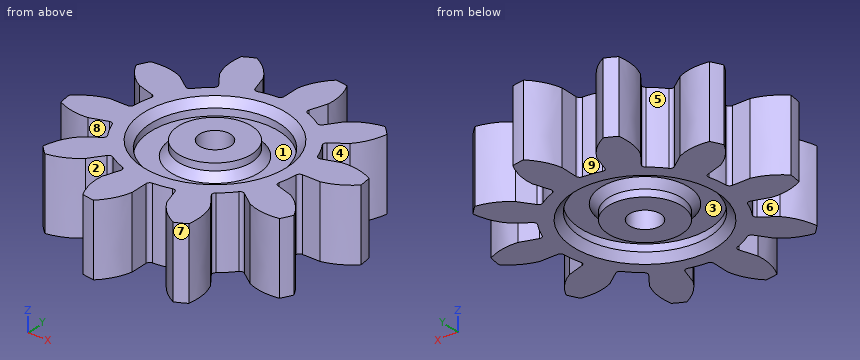
```python
from build123d import *

# Parameters (mm, degrees)
BOSS_EXTRUDE1_DEPTH = 10
CIRPATTERN1_COUNT   = 10
SKETCH1_R           = 11.7825
BOSS_EXTRUDE2_DEPTH = 10
SKETCH4_R           = 8.946052481
SKETCH4_R_2         = 5.101265003
CUT_EXTRUDE1_DEPTH  = 2
SKETCH4_3_R         = 2.163600103
CUT_EXTRUDE2_DEPTH  = 11.0000001
SKETCH5_R           = 8.946052481
SKETCH5_R_2         = 5.101265003
CUT_EXTRUDE3_DEPTH  = 2
FILLET1_R           = 0.5
CHAMFER1_SIZE       = 1
CHAMFER2_SIZE       = 1


with BuildPart() as part:
    # Sketch3 → Boss-Extrude1 (new body)
    with BuildSketch(Plane.XY):
        with BuildLine():
            Line((4.803075617, 13.959368513), (3.833494733, 11.141437267))
            ThreePointArc((3.833494733, 11.141437267), (1.943363276, 11.621129266), (0, 11.7825))
            Line((0, 11.7825), (0, 14.762571073))
            add(Edge.make_bspline(
                [(0, 14.762571073), (0.333518774, 16.315241106), (1.140884964, 17.626707575), (2.241097954, 18.718316804)],
                knots=[0, 0, 0, 0, 0.256830749, 0.256830749, 0.256830749, 0.256830749], degree=3))
            ThreePointArc((2.241097954, 18.718316804), (3.109381242, 18.593806826), (3.970932877, 18.429042191))
            add(Edge.make_bspline(
                [(4.803075617, 13.959368513), (4.992871831, 15.536072798), (4.656124965, 17.038865536), (3.970932877, 18.429042191)],
                knots=[0, 0, 0, 0, 0.256830749, 0.256830749, 0.256830749, 0.256830749], degree=3))
        make_face()
    extrude(amount=BOSS_EXTRUDE1_DEPTH)


with BuildPart() as cirpattern1_1:
    # CirPattern1: pattern copy
    add(part.part.rotate(Axis((0, 0, 0), (0, 0, 1)), 1 * 360 / CIRPATTERN1_COUNT))


with BuildPart() as cirpattern1_2:
    # CirPattern1: pattern copy
    add(part.part.rotate(Axis((0, 0, 0), (0, 0, 1)), 2 * 360 / CIRPATTERN1_COUNT))


with BuildPart() as cirpattern1_3:
    # CirPattern1: pattern copy
    add(part.part.rotate(Axis((0, 0, 0), (0, 0, 1)), 3 * 360 / CIRPATTERN1_COUNT))


with BuildPart() as cirpattern1_4:
    # CirPattern1: pattern copy
    add(part.part.rotate(Axis((0, 0, 0), (0, 0, 1)), 4 * 360 / CIRPATTERN1_COUNT))


with BuildPart() as cirpattern1_5:
    # CirPattern1: pattern copy
    add(part.part.rotate(Axis((0, 0, 0), (0, 0, 1)), 5 * 360 / CIRPATTERN1_COUNT))


with BuildPart() as cirpattern1_6:
    # CirPattern1: pattern copy
    add(part.part.rotate(Axis((0, 0, 0), (0, 0, 1)), 6 * 360 / CIRPATTERN1_COUNT))


with BuildPart() as cirpattern1_7:
    # CirPattern1: pattern copy
    add(part.part.rotate(Axis((0, 0, 0), (0, 0, 1)), 7 * 360 / CIRPATTERN1_COUNT))


with BuildPart() as cirpattern1_8:
    # CirPattern1: pattern copy
    add(part.part.rotate(Axis((0, 0, 0), (0, 0, 1)), 8 * 360 / CIRPATTERN1_COUNT))


with BuildPart() as cirpattern1_9:
    # CirPattern1: pattern copy
    add(part.part.rotate(Axis((0, 0, 0), (0, 0, 1)), 9 * 360 / CIRPATTERN1_COUNT))


with BuildPart() as part_1:
    add(part.part)

    add(cirpattern1_1.part)  # Boss-Extrude2 merges CirPattern1_1

    add(cirpattern1_2.part)  # Boss-Extrude2 merges CirPattern1_2

    add(cirpattern1_3.part)  # Boss-Extrude2 merges CirPattern1_3

    add(cirpattern1_4.part)  # Boss-Extrude2 merges CirPattern1_4

    add(cirpattern1_5.part)  # Boss-Extrude2 merges CirPattern1_5

    add(cirpattern1_6.part)  # Boss-Extrude2 merges CirPattern1_6

    add(cirpattern1_7.part)  # Boss-Extrude2 merges CirPattern1_7

    add(cirpattern1_8.part)  # Boss-Extrude2 merges CirPattern1_8

    add(cirpattern1_9.part)  # Boss-Extrude2 merges CirPattern1_9
    # Sketch1 → Boss-Extrude2 (add)
    with BuildSketch(Plane.XY):
        Circle(SKETCH1_R)
    extrude(amount=BOSS_EXTRUDE2_DEPTH)

    # Sketch4 → Cut-Extrude1 (cut)
    with BuildSketch(Plane.XY.offset(10)):
        Circle(SKETCH4_R)
        Circle(SKETCH4_R_2, mode=Mode.SUBTRACT)
    extrude(amount=-CUT_EXTRUDE1_DEPTH, mode=Mode.SUBTRACT)

    # Sketch4_3 → Cut-Extrude2 (cut, through all)
    with BuildSketch(Plane.XY.offset(10)):
        Circle(SKETCH4_3_R)
    extrude(amount=-CUT_EXTRUDE2_DEPTH, mode=Mode.SUBTRACT)

    # Sketch5 → Cut-Extrude3 (cut)
    with BuildSketch(Plane(origin=(0, 0, 0), x_dir=(-1, 0, 0), z_dir=(0, 0, -1))):
        Circle(SKETCH5_R)
        Circle(SKETCH5_R_2, mode=Mode.SUBTRACT)
    extrude(amount=-CUT_EXTRUDE3_DEPTH, mode=Mode.SUBTRACT)

    # Fillet1
    fillet1_edges = [part_1.edges().sort_by_distance(p)[0] for p in [
        (6.925579735, -9.532242736, 5),
        (3.447410128, -11.26688376, 5),
        (3.833494733, 11.141437267, 5),
        (0, 11.7825, 5),
        (11.205823403, -3.640992736, 5),
        (9.411521493, -7.088763604, 5),
        (11.205823403, 3.640992736, 5),
        (11.780751534, -0.202976689, 5),
        (6.925579735, 9.532242736, 5),
        (9.650134902, 6.760340422, 5),
        (-6.925579735, 9.532242736, 5),
        (-3.447410128, 11.26688376, 5),
        (-11.205823403, 3.640992736, 5),
        (-9.411521493, 7.088763604, 5),
        (-11.205823403, -3.640992736, 5),
        (-11.780751534, 0.202976689, 5),
        (-6.925579735, -9.532242736, 5),
        (-9.650134902, -6.760340422, 5),
        (0, -11.7825, 5),
        (-3.833494733, -11.141437267, 5),
    ]]
    fillet(fillet1_edges, radius=FILLET1_R)

    # Chamfer1
    chamfer1_edges = [part_1.edges().sort_by_distance(p)[0] for p in [
        (-5.101265003, 0, 8),
        (5.101265003, 0, 2),
    ]]
    chamfer(chamfer1_edges, length=CHAMFER1_SIZE)

    # Chamfer2
    chamfer2_edges = [part_1.edges().sort_by_distance(p)[0] for p in [
        (-8.946052481, 0, 10),
        (8.946052481, 0, 0),
    ]]
    chamfer(chamfer2_edges, length=CHAMFER2_SIZE)


solid = part_1.part
```
Geometry check sheet. Reference: the model listing, model coordinates, mm. Face numbers are marked on the shaded views. A direction names the side the tool comes from. Coordinates: 2 decimals unless noted, no trailing zeros. One line per item, written item: value. Start each with the question number.
(1) Mould release check, pull along Y, two halves, no side actions. Record for the marked faces 6, 7, 8 and 9: released by +Y, released by -Y, zero draft, split by the parting line, or undercut.
(2) Cross-section at A-A on z = 8.5. Count the separate pieces of the cut face and the enclosed holes in it, plus the area to 3 significant figures.
(3) Material ranges on line 1 (X direction, y = -13, z = 1.25); line 2 (Z direction, x = -3.5, y = 5); line 3 (X direction, y = 10.5, z = 6.5), recorded low to high. Write a range as [from, to].
(4) Depth check by flat-ended pin: P1, Ø5.5, axis at x = 0, y = 0, coming from the -Z side; P2, Ø2, axis at x = -6.5, z = 6.5, coming from the -Y side; P3, Ø2, axis at y = -14, z = 2.5, coming from the +X side; P4, Ø0.7, axis at y = 13.5, z = 7, coming from the -X side. Enter the tip coordinate at first touch or a pass-through.
(5) Tool access check on the marked faces 1, 2, 3, 4 and 5. Record the directions out of +Z, -Z, +X, -X, +Y, -Y that give a thin tool (end or side, any length) a straight path to the whole face; none if there is none.
Results below:
1. face 6: undercut
1. face 7: released by -Y
1. face 8: undercut
1. face 9: released by +Y
2. separate pieces: 2
2. enclosed holes: 2
2. area: 556 mm2
3. line 1: x = [-13.65, -10.21], [-4.47, 0], [3.98, 9.05]
3. line 2: z = [2, 8]
3. line 3: x = [-7.63, 5.35], [7.63, 13.43]
4. P1: stops at z = 0
4. P2: stops at y = -10.42
4. P3: stops at x = 9.31
4. P4: stops at x = -9.23
5. face 1: +Z
5. face 2: +Z, -Z, -Y
5. face 3: -Z
5. face 4: +Z, -Z, +X
5. face 5: +Z, -Z
